For this review, take the finished solid that the model builds, in its own axes (mm). Face numbers are marked on the shaded views. A direction names the side the tool comes from. Coordinates: 2 decimals unless noted, no trailing zeros. Loops run counter-clockwise (first coordinate to the right, second up) from the corner with the lowest first, then second, coordinate; pieces in that order, holes last.
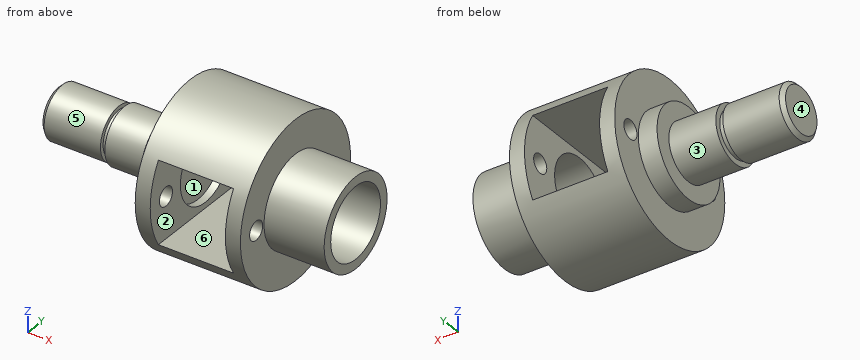
```python
from build123d import *

# Parameters (mm, degrees)
F_2_5_2_5_DIAMETER_HOLE1_D     = 2.5
CUT_EXTRUDE1_REACH             = 44.199
SKETCH3_W                      = 10
SKETCH3_H                      = 11
CUT_EXTRUDE1_DIRECTION_2_REACH = 44.199
CHAMFER1_SIZE                  = 0.5


with BuildPart() as part:
    # Sketch2 → Revolve1 (revolve)
    with BuildSketch(Plane.XY, mode=Mode.PRIVATE) as revolve1_sk:
        Polygon((0, 4.75), (0, 6), (-8, 6), (-8, 10.5), (-22, 10.5), (-22, 6), (-24.5, 6), (-24.5, 3.75), (-30.75, 3.75), (-30.75, 3), (-31.5, 3), (-31.5, 3.5), (-39.5, 3.5), (-39.5, 0), (-21, 0), (-21, 4.75), align=None)
    revolve(revolve1_sk.sketch.rotate(Axis((-21, 0, 0), (1, 0, 0)), 180), axis=Axis((-21, 0, 0), (1, 0, 0)))

    # Ø2.5 (2.5) Diameter Hole1 (through all)
    with Locations(Plane(origin=(-8, 0, 0), x_dir=(0, 0, -1), z_dir=(1, 0, 0))):
        with Locations((0, 7.5), (0, -7.5)):
            Hole(F_2_5_2_5_DIAMETER_HOLE1_D / 2)

    # Sketch3 → Cut-Extrude1 (cut, up to next)
    with BuildSketch(Plane(origin=(0, 0, 0), x_dir=(1, 0, 0), z_dir=(0, 1, 0)), mode=Mode.PRIVATE) as cut_extrude1_sk1:
        with Locations((-15, 0)):
            Rectangle(SKETCH3_W, SKETCH3_H)
    cut_extrude1_tool1 = extrude(cut_extrude1_sk1.sketch, amount=-CUT_EXTRUDE1_REACH, mode=Mode.PRIVATE) & part.part
    add(cut_extrude1_tool1.solids().sort_by_distance((-15, 0, 0))[0], mode=Mode.SUBTRACT)

    # Sketch3 → Cut-Extrude1 direction 2 (cut, up to next)
    with BuildSketch(Plane(origin=(0, 0, 0), x_dir=(1, 0, 0), z_dir=(0, 1, 0)), mode=Mode.PRIVATE) as cut_extrude1_direction_2_sk1:
        with Locations((-15, 0)):
            Rectangle(SKETCH3_W, SKETCH3_H)
    cut_extrude1_direction_2_tool1 = extrude(cut_extrude1_direction_2_sk1.sketch, amount=CUT_EXTRUDE1_DIRECTION_2_REACH, mode=Mode.PRIVATE) & part.part
    add(cut_extrude1_direction_2_tool1.solids().sort_by_distance((-15, 0, 0))[0], mode=Mode.SUBTRACT)

    # Chamfer1
    chamfer1_edges = [part.edges().sort_by_distance(p)[0] for p in [
        (-39.5, 3.5, 0),
    ]]
    chamfer(chamfer1_edges, length=CHAMFER1_SIZE)


solid = part.part
```
Q1. For pin 1 Ø11 at (x, y) = (-16.5, 3) entering from +Z; pin 2 Ø4 at (x, z) = (-8, -6.5) entering from -Y; pin 3 Ø4 at (y, z) = (-7.5, 0) entering from -X; pin 4 Ø6 at (x, z) = (-31, -1) entering from +Y, all flat-tipped, find the tip position at first contact; note any pin that passes through.
Q2. Consider section A-A (y = 8.25). State the section outline as (x, z) points, then the cut area to 3 significant figures.
Q3. Consider section C-C (y = -5.25). State the section outline as (x, z) points.
Q4. Machinability: for the marked faces 1, 2 and 3, which of the approach directions +Z, -Z, +X, -X, +Y, -Y give a long, thin tool a straight path to every point of the face, cutting with its end or side? Answer none if there is none.
Q5. Consider section B-B (x = -11). State the section outline as (y, z) points, then the cut area to 3 significant figures.
Q6. Wall thickness on probe 1 along Y at (x, z) = (-20.8, 0); probe 2 along X at (y, z) = (9.75, 0); probe 3 along Z at (x, y) = (-20.55, 0): over which ranges is each line inside the solid? List them lowest first.
Q7. Consider section D-D (z = 0). Count the separate pieces of the cut face and the enclosed holes in it, then the cut area to 3 significant figures.
Q8. The part is to be moulded in two halves that separate along X. For the marked faces 4, 5 and 6, say which applies: +X half, -X half, draft (parallel to the pull), parting line (faces both ways), or undercut.
Model answer:
1. pin 1: stops at z = 10.5
1. pin 2: stops at y = -9.49
1. pin 3: stops at x = -24.5
1. pin 4: stops at y = 3.75
2. outline: (-22, -6.5) - (-8, -6.5) - (-8, -1) - (-10, -1) - (-10, -5.5) - (-20, -5.5) - (-20, -1) - (-22, -1) - close; (-22, 1) - (-20, 1) - (-20, 5.5) - (-10, 5.5) - (-10, 1) - (-8, 1) - (-8, 6.5) - (-22, 6.5) - close
2. area: 63.9 mm2
3. outline: (-24.5, -2.9) - (-22, -2.9) - (-22, -9.09) - (-8, -9.09) - (-8, -2.9) - (0, -2.9) - (0, 2.9) - (-8, 2.9) - (-8, 9.09) - (-22, 9.09) - (-22, 2.9) - (-24.5, 2.9) - close; hole (-20, -5.5) - (-10, -5.5) - (-10, 5.5) - (-20, 5.5) - close
4. face 1: +X
4. face 2: +Y, -Y
4. face 3: -X
5. outline: (-8.94, -5.5) arc R10.5 ccw to (8.94, -5.5) - close; (-8.94, 5.5) - (8.94, 5.5) arc R10.5 ccw to start
5. area: 126 mm2
6. probe 1: y = -10.5 to -8.75, -6.25 to -4.75, 4.75 to 6.25, 8.75 to 10.5
6. probe 2: x = -22 to -20, -10 to -8
6. probe 3: z = -10.5 to -4.75, 4.75 to 10.5
7. separate pieces: 7
7. enclosed holes: 0
7. area: 193 mm2
8. face 4: -X half
8. face 5: draft
8. face 6: undercut
